```python
from build123d import *

# Parameters (mm, degrees)
SKETCH1_W               = 355.6
SKETCH1_H               = 279.4
BOSS_EXTRUDE1_DEPTH     = 3.175
F_1_4_CLEARANCE_HOLE1_D = 7.14248
CUT_EXTRUDE1_REACH      = 454.245
SKETCH4_R               = 254


with BuildPart() as part:
    # Sketch1 → Boss-Extrude1 (new body)
    with BuildSketch(Plane.XY):
        with Locations((177.8, -139.7)):
            Rectangle(SKETCH1_W, SKETCH1_H)
    extrude(amount=BOSS_EXTRUDE1_DEPTH)

    # 1/4 Clearance Hole1 (through all)
    with Locations(Plane.XY.offset(3.175)):
        with Locations((342.9, -63.5), (342.9, -266.7), (12.7, -266.7), (12.7, -63.5)):
            Hole(F_1_4_CLEARANCE_HOLE1_D / 2)

    # Sketch4 → Cut-Extrude1 (cut, up to next)
    with BuildSketch(Plane.XY.offset(3.175), mode=Mode.PRIVATE) as cut_extrude1_sk1:
        with Locations((177.8, 177.8)):
            Circle(SKETCH4_R)
    cut_extrude1_tool1 = extrude(cut_extrude1_sk1.sketch, amount=-CUT_EXTRUDE1_REACH, mode=Mode.PRIVATE) & part.part
    add(cut_extrude1_tool1.solids().sort_by_distance((177.8, 177.8, 3.175))[0], mode=Mode.SUBTRACT)


solid = part.part
```
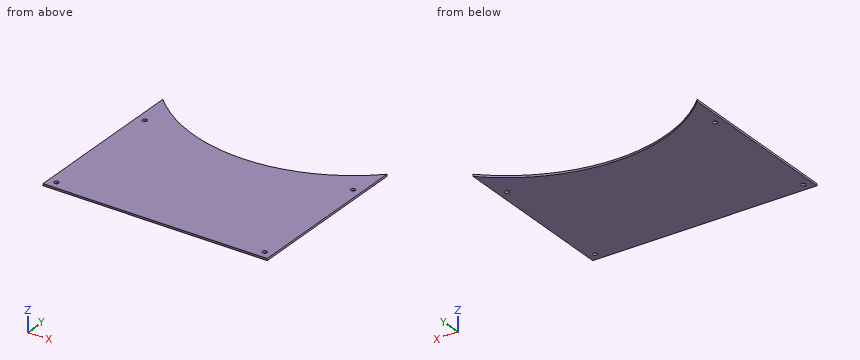
Read the model definition and answer for the solid it produces. Units are mm, in the model's axes. Coordinates: 2 decimals unless noted, no trailing zeros. Write each loop counter-clockwise with the first axis right and the second up, starting at its lowest first coordinate (ties: lowest second). Pieces come first, ordered by that corner, then holes. Notation, with made-up numbers: (14.5, -2) -> (19.5, -2) arc R6 ccw to (19.5, 2) -> close; hole circle Ø5 at (54, -2.5). An arc over 180 degrees is marked (long way). Write item = value, one per line.
(1) Straight lines are drawn through the part: L1, parallel to X at y = -266.7, z = 2.05; L2, parallel to Y at x = 342.9, z = 1.05; L3, parallel to Y at x = 180.5, z = 0.25. For each, find the intervals that lie inside material, in ascending order. Write a range as from..to.
From the geometry:
L1 = 0..9.13, 16.27..339.33, 346.47..355.6
L2 = -279.4..-270.27, -263.13..-67.07, -59.93..-15.22
L3 = -279.4..-76.19
(2) Section C-C on x = 269.5 is taken. Write down the section's boundary in (y, z) (3 decimals), plus the area to 3 significant figures.
From the geometry:
outline = (-279.4, 0) -> (-59.069, 0) -> (-59.069, 3.175) -> (-279.4, 3.175) -> close
area = 700 mm2
(3) Section A-A on z = 0.5 is taken. Write down the section's boundary in (x, y).
From the geometry:
outline = (0, -279.4) -> (355.6, -279.4) -> (355.6, -3.59) arc R254 cw to (0, -3.59) -> close; hole circle Ø7.14 at (12.7, -266.7); hole circle Ø7.14 at (12.7, -63.5); hole circle Ø7.14 at (342.9, -266.7); hole circle Ø7.14 at (342.9, -63.5)
(4) Section B-B on x = 111 is taken. Write down the section's boundary in (y, z) (3 decimals), plus the area to 3 significant figures.
From the geometry:
outline = (-279.4, 0) -> (-67.259, 0) -> (-67.259, 3.175) -> (-279.4, 3.175) -> close
area = 674 mm2
(5) Given pin 1 Ø3 at (x, y) = (288.5, -217) entering from -Z, flat-ended and moving along its own axis, determine where the tip first touches the part or whether it passes through.
From the geometry:
pin_1 = 0
